Input: part model. Units: mm. Frame: model coordinates. A direction names the side the tool comes from. Round coordinates to 2 decimals unless told otherwise and drop trailing zeros. Loops run counter-clockwise (first coordinate to the right, second up) from the corner with the lowest first, then second, coordinate; pieces in that order, holes last. Notation, with made-up numbers: (86.5, 19) - (109.5, 19) arc R18 cw to (109.5, 27) - close; hole circle Ø6 at (-22.5, 30.5). An arc over 180 degrees is marked (long way). Write each question's results on one line, items separated by ' | '.
from build123d import *

# Parameters (mm, degrees)
BOSS_EXTRUDE1_DEPTH                     = 56
SKETCH2_W                               = 32
SKETCH2_H                               = 74
CUT_EXTRUDE1_DEPTH                      = 56
CHAMFER1_SIZE                           = 2
CBORE_FOR_M6_HEX_HEAD_BOLT1_D           = 10
CBORE_FOR_M6_HEX_HEAD_BOLT1_DEPTH       = 20
CBORE_FOR_M6_HEX_HEAD_BOLT1_CBORE_D     = 12
CBORE_FOR_M6_HEX_HEAD_BOLT1_CBORE_DEPTH = 4
CBORE_FOR_M6_HEX_HEAD_BOLT1_TIP         = 3.004303095
CBORE_FOR_M6_HEX_HEAD_BOLT3_D           = 10
CBORE_FOR_M6_HEX_HEAD_BOLT3_DEPTH       = 20
CBORE_FOR_M6_HEX_HEAD_BOLT3_CBORE_D     = 12
CBORE_FOR_M6_HEX_HEAD_BOLT3_CBORE_DEPTH = 4
CBORE_FOR_M6_HEX_HEAD_BOLT3_TIP         = 3.004303095
M6X1_0_TAPPED_HOLE1_D                   = 5
M6X1_0_TAPPED_HOLE1_DEPTH               = 27
M6X1_0_TAPPED_HOLE1_TIP                 = 1.502151548


with BuildPart() as part:
    # Sketch1 → Boss-Extrude1 (new body)
    with BuildSketch(Plane.XY):
        Polygon((0, 0), (12.5, 0), (12.5, 45), (7.5, 84), (-7.5, 84), (-12.5, 45), (-12.5, 0), align=None)
    extrude(amount=BOSS_EXTRUDE1_DEPTH)

    # Sketch2 → Cut-Extrude1 (cut)
    with BuildSketch(Plane(origin=(12.5, 0, 0), x_dir=(0, 0, -1), z_dir=(1, 0, 0))):
        with Locations((-28, 47)):
            Rectangle(SKETCH2_W, SKETCH2_H)
    extrude(amount=-CUT_EXTRUDE1_DEPTH, mode=Mode.SUBTRACT)

    # Chamfer1
    chamfer1_edges = [part.edges().sort_by_distance(p)[0] for p in [
        (-12.5, 10, 28),
        (12.5, 10, 28),
    ]]
    chamfer(chamfer1_edges, length=CHAMFER1_SIZE)

    # CBORE for M6 Hex Head Bolt1
    with Locations(Plane.XY.offset(56)):
        with Locations((0, 75)):
            CounterBoreHole(CBORE_FOR_M6_HEX_HEAD_BOLT1_D / 2, CBORE_FOR_M6_HEX_HEAD_BOLT1_CBORE_D / 2, CBORE_FOR_M6_HEX_HEAD_BOLT1_CBORE_DEPTH, depth=CBORE_FOR_M6_HEX_HEAD_BOLT1_DEPTH)
            with Locations((0, 0, -(CBORE_FOR_M6_HEX_HEAD_BOLT1_DEPTH + CBORE_FOR_M6_HEX_HEAD_BOLT1_TIP / 2))):  # 118° drill point
                Cone(0, CBORE_FOR_M6_HEX_HEAD_BOLT1_D / 2, CBORE_FOR_M6_HEX_HEAD_BOLT1_TIP, mode=Mode.SUBTRACT)

    # CBORE for M6 Hex Head Bolt3
    with Locations(Plane(origin=(0, 0, 0), x_dir=(-1, 0, 0), z_dir=(0, 0, -1))):
        with Locations((0, 75)):
            CounterBoreHole(CBORE_FOR_M6_HEX_HEAD_BOLT3_D / 2, CBORE_FOR_M6_HEX_HEAD_BOLT3_CBORE_D / 2, CBORE_FOR_M6_HEX_HEAD_BOLT3_CBORE_DEPTH, depth=CBORE_FOR_M6_HEX_HEAD_BOLT3_DEPTH)
            with Locations((0, 0, -(CBORE_FOR_M6_HEX_HEAD_BOLT3_DEPTH + CBORE_FOR_M6_HEX_HEAD_BOLT3_TIP / 2))):  # 118° drill point
                Cone(0, CBORE_FOR_M6_HEX_HEAD_BOLT3_D / 2, CBORE_FOR_M6_HEX_HEAD_BOLT3_TIP, mode=Mode.SUBTRACT)

    # M6x1.0 Tapped Hole1
    with Locations(Plane(origin=(0, 20, 0), x_dir=(-1, 0, 0), z_dir=(0, 0, -1))):
        with Locations((0, 0)):
            Hole(M6X1_0_TAPPED_HOLE1_D / 2, depth=M6X1_0_TAPPED_HOLE1_DEPTH)
            with Locations((0, 0, -(M6X1_0_TAPPED_HOLE1_DEPTH + M6X1_0_TAPPED_HOLE1_TIP / 2))):  # 118° drill point
                Cone(0, M6X1_0_TAPPED_HOLE1_D / 2, M6X1_0_TAPPED_HOLE1_TIP, mode=Mode.SUBTRACT)


solid = part.part
1. Set-up query: faces 1 (the flat face through (-11.5, 9, 28.2)), 2 (the flat face through (-9.965, 64.773, 5.916)), 3 (the cylindrical face through (0.78, 80.95, 1.97)), 4 (the flat face through (-4, 79, 52)), 5 (the flat face through (-12.5, 7.8, 27.6)). Return all of +Z, -Z, +X, -X, +Y, -Y with unobstructed straight access to the full face (end or side cutting, diameter ignored); none if empty.
Answer:
face 1: -X, +Y | face 2: +Z, -Z, -X, +Y | face 3: -Z | face 4: +Z | face 5: +Z, -Z, -X, +Y, -Y
2. Section query C-C, the plane y = 20. Output: boundary loops of the cut face in (x, z).
Answer:
outline: (-12.5, 0) - (-2.5, 0) - (-2.5, 12) - (-12.5, 12) - close; (-12.5, 44) - (12.5, 44) - (12.5, 56) - (-12.5, 56) - close; (2.5, 0) - (12.5, 0) - (12.5, 12) - (2.5, 12) - close
3. Line query: line 1 (Y direction, x = 0, z = 7.5); line 2 (Z direction, x = -4, y = 36); line 3 (Y direction, x = 0, z = 1.7). Output: solid intervals per line, ascending. Write a range as [from, to].
Answer:
line 1: [0, 17.5], [22.5, 70], [80, 84] | line 2: [0, 12], [44, 56] | line 3: [0, 17.5], [22.5, 69], [81, 84]
4. Mould query, pull axis Z, two halves, no side actions, for faces 6 (the flat face through (0, 33, 0)), 7 (the flat face through (0, 10, 28)), 8 (the flat face through (11.5, 9, 28.2)), 9 (the flat face through (0, 0, 28)). Classes: pulls with the +Z half, pulls with the -Z half, needs draft (parallel to the pull), parting line crosses it, or undercut.
Answer:
face 6: pulls with the -Z half | face 7: undercut | face 8: undercut | face 9: needs draft
5. Section query A-A, the plane y = 64.5. Output: boundary loops of the cut face in (x, z).
Answer:
outline: (-10, 0) - (10, 0) - (10, 12) - (-10, 12) - close; (-10, 44) - (10, 44) - (10, 56) - (-10, 56) - close
6. Section query D-D, the plane z = 17. Output: boundary loops of the cut face in (x, y), plus the area to 3 significant figures.
Answer:
outline: (-12.5, 0) - (12.5, 0) - (12.5, 8) - (10.5, 10) - (-10.5, 10) - (-12.5, 8) - close | area: 246 mm^2
7. Section query B-B, the plane x = 0. Output: boundary loops of the cut face in (y, z), plus the area to 3 significant figures.
Answer:
outline: (0, 0) - (17.5, 0) - (17.5, 12) - (10, 12) - (10, 44) - (70, 44) - (70, 52) - (69, 52) - (69, 56) - (0, 56) - close; (22.5, 0) - (69, 0) - (69, 4) - (70, 4) - (70, 12) - (22.5, 12) - close; (80, 4) - (81, 4) - (81, 0) - (84, 0) - (84, 12) - (80, 12) - close; (80, 44) - (84, 44) - (84, 56) - (81, 56) - (81, 52) - (80, 52) - close | area: 2,020 mm^2
8. Contact query for flat-ended pins moving along their axis: pin 1 (11.5 mm diameter, centred on x = 0, y = 75, fed in from -Z); pin 2 (11 mm diameter, centred on x = 0, y = 75, fed in from +Z); pin 3 (6.5 mm diameter, centred on x = -4, z = 30, fed in from +Y). Output: stop coordinate, or through.
Answer:
pin 1: z = 4 | pin 2: z = 52 | pin 3: y = 10
